```python
from build123d import *

# Parameters (mm, degrees)
SKETCH_1_W          = 80
SKETCH_1_H          = 50
EXTRUDE_1_DEPTH     = 1.6
SKETCH_2_R          = 1.55
CUT_EXTRUDE_1_DEPTH = 2.6
SKETCH_3_W          = 6
SKETCH_3_H          = 6
EXTRUDE_2_DEPTH     = 3.5
SKETCH_4_R          = 1.75
EXTRUDE_3_DEPTH     = 4.5
SKETCH_5_W          = 12
SKETCH_5_H          = 12
EXTRUDE_4_DEPTH     = 3
SKETCH_6_W          = 10
SKETCH_6_H          = 10
EXTRUDE_5_DEPTH     = 2
SKETCH_7_W          = 16
SKETCH_7_H          = 18
SKETCH_7_W_2        = 3
SKETCH_7_H_2        = 4
SKETCH_7_W_3        = 5
SKETCH_7_H_3        = 10.5
SKETCH_7_W_4        = 8
SKETCH_7_W_5        = 10.5
SKETCH_7_H_4        = 21.5
SKETCH_7_W_6        = 7.5
SKETCH_7_H_5        = 7
SKETCH_7_W_7        = 9
SKETCH_7_H_6        = 5
SKETCH_7_W_8        = 4
SKETCH_7_H_7        = 3
EXTRUDE_6_DEPTH     = 3
SKETCH_8_W          = 6.5
SKETCH_8_H          = 8
EXTRUDE_7_DEPTH     = 5
SKETCH_9_W          = 15
SKETCH_9_H          = 9
EXTRUDE_8_DEPTH     = 11


with BuildPart() as part:
    # ｽｹｯﾁ1 → ﾎﾞｽ - 押し出し1 (new body)
    with BuildSketch(Plane.XY):
        with Locations((40, 25)):
            Rectangle(SKETCH_1_W, SKETCH_1_H)
    extrude(amount=EXTRUDE_1_DEPTH)

    # ｽｹｯﾁ2 → ｶｯﾄ - 押し出し1 (cut, through all)
    with BuildSketch(Plane.XY.offset(1.6)):
        with Locations((75, 45)):
            Circle(SKETCH_2_R)
        with Locations((75, 5)):
            Circle(SKETCH_2_R)
        with Locations((5, 5)):
            Circle(SKETCH_2_R)
        with Locations((5, 45)):
            Circle(SKETCH_2_R)
    extrude(amount=-CUT_EXTRUDE_1_DEPTH, mode=Mode.SUBTRACT)

    # ｽｹｯﾁ3 → ﾎﾞｽ - 押し出し2 (add)
    with BuildSketch(Plane.XY.offset(1.6)):
        with Locations((60, 14)):
            Rectangle(SKETCH_3_W, SKETCH_3_H)
        with Locations((20, 14)):
            Rectangle(SKETCH_3_W, SKETCH_3_H)
    extrude(amount=EXTRUDE_2_DEPTH)

    # ｽｹｯﾁ4 → ﾎﾞｽ - 押し出し3 (add)
    with BuildSketch(Plane.XY.offset(5.1)):
        with Locations((20, 14)):
            Circle(SKETCH_4_R)
        with Locations((60, 14)):
            Circle(SKETCH_4_R)
    extrude(amount=EXTRUDE_3_DEPTH)

    # ｽｹｯﾁ5 → ﾎﾞｽ - 押し出し4 (add)
    with BuildSketch(Plane.XY.offset(1.6)):
        with Locations((40, 12)):
            Rectangle(SKETCH_5_W, SKETCH_5_H)
    extrude(amount=EXTRUDE_4_DEPTH)

    # ｽｹｯﾁ6 → ﾎﾞｽ - 押し出し5 (add)
    with BuildSketch(Plane.XY.offset(1.6)):
        with Locations((69, 35)):
            Rectangle(SKETCH_6_W, SKETCH_6_H)
    extrude(amount=EXTRUDE_5_DEPTH)

    # ｽｹｯﾁ7 → ﾎﾞｽ - 押し出し6 (add)
    with BuildSketch(Plane(origin=(0, 0, 0), x_dir=(-1, 0, 0), z_dir=(0, 0, -1))):
        with Locations((-21, 34)):
            Rectangle(SKETCH_7_W, SKETCH_7_H)
        with Locations((-5, 27)):
            Rectangle(SKETCH_7_W_2, SKETCH_7_H_2)
        with Locations((-19, -0.25)):
            Rectangle(SKETCH_7_W_3, SKETCH_7_H_3)
        with Locations((-55, -0.25)):
            Rectangle(SKETCH_7_W_4, SKETCH_7_H_3)
        with Locations((-74.75, 19.25)):
            Rectangle(SKETCH_7_W_5, SKETCH_7_H_4)
        with Locations((-60.25, 48)):
            Rectangle(SKETCH_7_W_6, SKETCH_7_H_5)
        with Locations((-47.7, 42)):
            Rectangle(SKETCH_7_W_7, SKETCH_7_H_6)
        with Locations((-40, 39.5)):
            Rectangle(SKETCH_7_W_8, SKETCH_7_H_7)
        with Locations((-61, 27)):
            Rectangle(SKETCH_7_W_3, SKETCH_7_H_2)
    extrude(amount=EXTRUDE_6_DEPTH)

    # ｽｹｯﾁ8 → ﾎﾞｽ - 押し出し7 (add)
    with BuildSketch(Plane(origin=(0, 0, 0), x_dir=(-1, 0, 0), z_dir=(0, 0, -1))):
        with Locations((-39.85, 30.5)):
            Rectangle(SKETCH_8_W, SKETCH_8_H)
    extrude(amount=EXTRUDE_7_DEPTH)

    # ｽｹｯﾁ9 → ﾎﾞｽ - 押し出し8 (add)
    with BuildSketch(Plane(origin=(0, 0, 0), x_dir=(-1, 0, 0), z_dir=(0, 0, -1))):
        with Locations((-72.5, 37)):
            Rectangle(SKETCH_9_W, SKETCH_9_H)
    extrude(amount=EXTRUDE_8_DEPTH)


solid = part.part
```
Geometry: final body of the model. Coordinates: model frame, mm. A direction names the side the tool comes from. Give positions to 0.01 mm unless a question says otherwise; leave off trailing zeros. Order: outer loops, then holes, each group sorted by start corner. A loop starts at its lowest first (then second) coordinate and runs counter-clockwise, first axis right, second up. Notation, with made-up numbers: (-10.75, -0.5) -> (6.25, -0.5) arc R12 ccw to (6.25, 4.5) -> close; hole circle Ø9 at (22.25, -14.5). An arc over 180 degrees is marked (long way). Write each question's results on one line, items separated by ' | '. Start each with the question number.
1) Set-up query: faces 1 (the flat face through (64, 48, -1)), 2 (the flat face through (38, 39, -1)), 3 (the flat face through (60, 44.5, -1)). Return all of +Z, -Z, +X, -X, +Y, -Y with unobstructed straight access to the full face (end or side cutting, diameter ignored); none if empty.
2) First-contact query: pin 1 (8 mm diameter, centred on x = 48, y = 7, fed in from +Z); pin 2 (1.7 mm diameter, centred on x = 19.5, z = 3, fed in from +Y); pin 3 (1 mm diameter, centred on x = 58.5, z = 3, fed in from -Y); pin 4 (6 mm diameter, centred on x = 48.5, z = 1.5, fed in from -Y). Flat tips, straight axial feed; report the tip coordinate or a pass-through.
3) Line query: line 1 (Y direction, x = 5, z = 1.15); line 2 (X direction, y = 27.5, z = -1); line 3 (X direction, y = -3, z = -0.5). Output: solid intervals per line, ascending. Write a range as from..to.
4) Section C-C (x = 60). Return loops of the section in (y, z).
5) Section A-A (x = 75). Return loops of the section in (y, z), then the cut area to 3 significant figures.
6) Draft query along Y for faces 4 (the flat face through (20, 17, 3)), 5 (the cylindrical face through (3.45, 5.07, 0.81)), 6 (the flat face through (55, 0, -3)). Return one class per face: pulls with the +Y half, pulls with the -Y half, needs draft (parallel to the pull), parting line crosses it, or undercut.
7) Section D-D (y = 21). Return loops of the section in (x, z), then the cut area to 4 significant figures.
8) Section B-B (z = -1.5). Count the separate pieces of the cut face and the enclosed holes in it, then the cut area to 3 significant figures.
Calculated:
1) face 1: -Z, +X, +Y, -Y | face 2: -Z, +Y | face 3: -Z, +X
2) pin 1: z = 4.6 | pin 2: y = 17 | pin 3: y = 11 | pin 4: y = -5.5
3) line 1: 0..3.45, 6.55..43.45, 46.55..50 | line 2: 3.5..6.5, 13..29, 36.6..43.1, 58.5..63.5, 69.5..80 | line 3: 16.5..21.5, 51..59
4) outline: (0, 0) -> (25, 0) -> (25, -3) -> (29, -3) -> (29, 0) -> (44.5, 0) -> (44.5, -3) -> (51.5, -3) -> (51.5, 0) -> (50, 0) -> (50, 1.6) -> (17, 1.6) -> (17, 5.1) -> (15.75, 5.1) -> (15.75, 9.6) -> (12.25, 9.6) -> (12.25, 5.1) -> (11, 5.1) -> (11, 1.6) -> (0, 1.6) -> close
5) outline: (0, 0) -> (3.45, 0) -> (3.45, 1.6) -> (0, 1.6) -> close; (6.55, 0) -> (8.5, 0) -> (8.5, -3) -> (30, -3) -> (30, 0) -> (32.5, 0) -> (32.5, -11) -> (41.5, -11) -> (41.5, 0) -> (43.45, 0) -> (43.45, 1.6) -> (6.55, 1.6) -> close; (46.55, 0) -> (50, 0) -> (50, 1.6) -> (46.55, 1.6) -> close | area: 234 mm2
6) face 4: pulls with the +Y half | face 5: undercut | face 6: needs draft
7) outline: (0, 0) -> (69.5, 0) -> (69.5, -3) -> (80, -3) -> (80, 1.6) -> (0, 1.6) -> close | area: 159.5 mm2
8) separate pieces: 11 | enclosed holes: 0 | area: 979 mm2
